Source: CAD feature listing. Evaluate the final solid. Frame: model axes, mm. Face numbers are marked on the shaded views. A direction names the side the tool comes from. Give positions to 0.01 mm unless a question says otherwise; leave off trailing zeros. Order: outer loops, then holes, each group sorted by start corner. A loop starts at its lowest first (then second) coordinate and runs counter-clockwise, first axis right, second up.
```python
from build123d import *

# Parameters (mm, degrees)
SCHIZZO1_W               = 25
SCHIZZO1_H               = 21.5
ESTRUSIONE1_DEPTH        = 85
SCHIZZO6_W               = 73
SCHIZZO6_H               = 23.639461627
TAGLIO_ESTRUSIONE4_DEPTH = 84
SCHIZZO7_R               = 5.5
ESTRUSIONE4_DEPTH        = 73
SMUSSO1_SIZE             = 0.803847577
SMUSSO1_SIZE_2           = 3
SCHIZZO8_R               = 3
TAGLIO_ESTRUSIONE5_DEPTH = 8.5


with BuildPart() as part:
    # Schizzo1 → Estrusione1 (new body)
    with BuildSketch(Plane.XY):
        with Locations((12.5, 10.75)):
            Rectangle(SCHIZZO1_W, SCHIZZO1_H)
    extrude(amount=ESTRUSIONE1_DEPTH)

    # Schizzo6 → Taglio-Estrusione4 (cut)
    with BuildSketch(Plane(origin=(25, 0, 0), x_dir=(0, 0, -1), z_dir=(1, 0, 0))):
        with Locations((-42.5, 20.319730814)):
            Rectangle(SCHIZZO6_W, SCHIZZO6_H)
    extrude(amount=-TAGLIO_ESTRUSIONE4_DEPTH, mode=Mode.SUBTRACT)

    # Schizzo7 → Estrusione4 (add)
    with BuildSketch(Plane.XY.offset(6)):
        with Locations(Location((6, 17, 0), (0, 0, 125.096801228))):
            Circle(SCHIZZO7_R)
        with Locations(Location((18.5, 17, 0), (0, 0, 125.096801228))):
            Circle(SCHIZZO7_R)
    extrude(amount=ESTRUSIONE4_DEPTH)

    # Smusso1
    # the kernel refuses this chamfer: 3, 0.803847577 mm, written as the material it takes off along each edge
    with BuildSketch(Plane(origin=(0, 21.5, -7.790164711), x_dir=(-0.13751244702128895, -0.9905000388259545, 0), z_dir=(0, 0, 1)), Plane(origin=(0, 21.5, 79), x_dir=(-0.13751244702128895, -0.9905000388259545, 0), z_dir=(0, 0, 1))) as smusso1_piece_1:
        Polygon((SMUSSO1_SIZE * 0.990500039187, SMUSSO1_SIZE * 0.137512447071), (-SMUSSO1_SIZE_2 * 0.137512447021, SMUSSO1_SIZE_2 * 0.990500038826), (0, 0), align=None)
    extrude(amount=13.790164711, mode=Mode.SUBTRACT)
    with BuildSketch(Plane(origin=(25, 21.5, -7.790164711), x_dir=(0.13751244702128734, -0.9905000388259546, 0), z_dir=(0, 0, 1)), Plane(origin=(25, 21.5, 71.209835289), x_dir=(0.13751244702128734, -0.9905000388259546, 0), z_dir=(0, 0, 1))) as smusso1_piece_2:
        Polygon((SMUSSO1_SIZE * 0.990500039187, -SMUSSO1_SIZE * 0.137512447071), (-SMUSSO1_SIZE_2 * 0.137512447021, -SMUSSO1_SIZE_2 * 0.990500038826), (0, 0), align=None)
    extrude(amount=21.580329421, mode=Mode.SUBTRACT)

    # Schizzo8 → Taglio-Estrusione5 (cut)
    with BuildSketch(Plane.XZ):
        with Locations(Location((12, 75.5, 0), (0, 0, 270))):
            Circle(SCHIZZO8_R)
        with Locations(Location((12, 9.5, 0), (0, 0, 270))):
            Circle(SCHIZZO8_R)
    extrude(amount=-TAGLIO_ESTRUSIONE5_DEPTH, mode=Mode.SUBTRACT)


solid = part.part
```
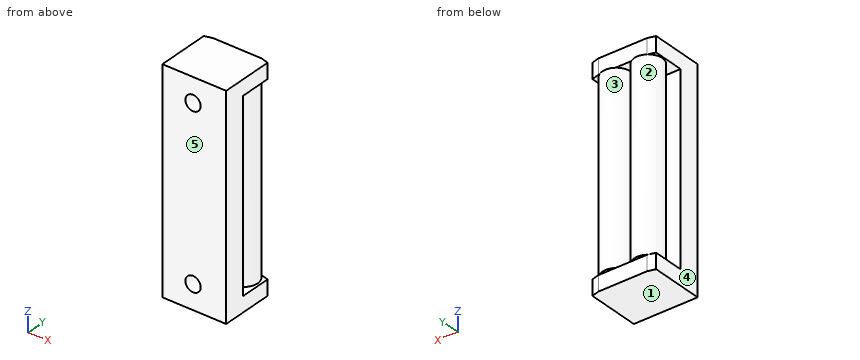
1) Pin query (flat end, axial travel): pin 1 (5 mm diameter, centred on x = 12, z = 75.5, fed in from +Y); pin 2 (1.8 mm diameter, centred on x = 10, z = 2.5, fed in from +Y); pin 3 (0.5 mm diameter, centred on x = 19, y = 22, fed in from -Z); pin 4 (5 mm diameter, centred on x = 15, y = 6.5, fed in from -Z). Return the tip coordinate at first contact, or that it passes through.
Report:
pin 1: stops at y = 21.24
pin 2: stops at y = 21.5
pin 3: stops at z = 6
pin 4: stops at z = 0
2) Section query C-C, the plane z = 75.5. Return the cut outline in (x, y).
Report:
outline: (0, 0) - (9, 0) - (9, 8.5) - (0, 8.5) - close; circle Ø11 at (6, 17); circle Ø11 at (18.5, 17); (15, 0) - (25, 0) - (25, 8.5) - (15, 8.5) - close
3) Material intervals for L1, parallel to Y at x = 5.75, z = 14.5; L2, parallel to Z at x = 6.5, y = 9.5; L3, parallel to X at y = 6.75, z = 9.5, sorted ascending.
Report:
L1: y = 0 to 8.5, 11.51 to 22.49
L2: z = 0 to 6, 79 to 85
L3: x = 0 to 9, 15 to 25
4) Section query A-A, the plane y = 17. Return the cut outline in (x, z).
Report:
outline: (0, 0) - (25, 0) - (25, 6) - (24, 6) - (24, 79) - (25, 79) - (25, 85) - (0, 85) - (0, 79) - (0.5, 79) - (0.5, 6) - (0, 6) - close; hole (11.5, 6) - (13, 6) - (13, 79) - (11.5, 79) - close
5) Draft query along X for the marked faces 3, 4 and 5. Return one class per face: +X half, -X half, draft (parallel to the pull), parting line (faces both ways), or undercut.
Report:
face 3: undercut
face 4: -X half
face 5: draft
6) Section query B-B, the plane x = 6. Return the cut outline in (y, z), and give its area (3 significant figures).
Report:
outline: (0, 0) - (21.5, 0) - (21.5, 6) - (22.5, 6) - (22.5, 79) - (21.5, 79) - (21.5, 85) - (0, 85) - close; hole (8.5, 6) - (11.5, 6) - (11.5, 79) - (8.5, 79) - close
area: 1,680 mm2
7) Reachability of the marked faces 1 and 2 from +Z, -Z, +X, -X, +Y, -Y: full face, straight path, thin tool, end or side. Return the list, or none.
Report:
face 1: -Z, +X, -X, +Y, -Y
face 2: none
8) Section query D-D, the plane y = 4. Return the cut outline in (x, z).
Report:
outline: (0, 0) - (25, 0) - (25, 85) - (0, 85) - close; hole circle Ø6 at (12, 9.5); hole circle Ø6 at (12, 75.5)
